Build history of the part. All positions in model axes, mm. Face numbers are marked on the shaded views. A direction names the side the tool comes from. Give positions to 0.01 mm unless a question says otherwise; leave off trailing zeros. Order: outer loops, then holes, each group sorted by start corner. A loop starts at its lowest first (then second) coordinate and runs counter-clockwise, first axis right, second up. Notation, with made-up numbers: (46, -39.5) -> (103, -39.5) arc R20 cw to (103, -24.5) -> close; hole circle Ø10 at (75.5, 61). An arc over 180 degrees is marked (long way). Write item = value, one per line. Start each with the question number.
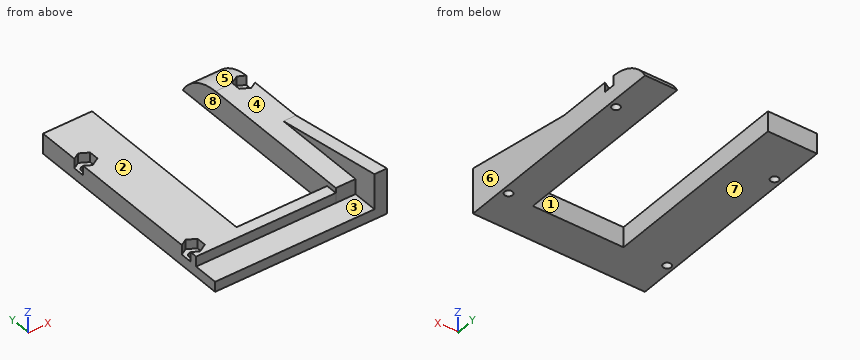
Autodesk Inventor part; units mm, degrees
ref_plane "Work Plane1" through (0, 0, 2.5241) normal (0, 0, 1) x (1, 0, 0)
ref_plane "YZ Plane" through (0, 0, 0) normal (1, 0, 0) x (0, 1, 0)
ref_plane "XZ Plane" through (0, 0, 0) normal (0, 1, 0) x (-1, 0, 0)
ref_plane "Work Plane1" through (0, 0, 2.5241) normal (0, 0, 1) x (1, 0, 0)
sketch "Sketch1" plane through (0, 0, 2.5241) normal (0, 0, 1) x (1, 0, 0)
  line L0 (-4, 272) -> (-4, -8) construction
  line L1 (4, 272) -> (4, -8) construction
  line L2 (76, 272) -> (76, -8) construction
  line L3 (84, 272) -> (84, -8) construction
  line L4 (84, -8) -> (-4, -8) construction
  line L5 (84, 106) -> (80, 106) construction
  line L6 (80, 110) -> (76, 110) construction
  line L7 (-3.365, 272) -> (-3.365, -7.365) construction
  line L8 (-3.365, -7.365) -> (83.365, -7.365) construction
  line L9 (83.365, -7.365) -> (83.365, 272) construction
  line L10 (-3.365, -7.365) -> (83.365, -7.365)
  line L11 (83.365, -7.365) -> (83.365, 107.95)
  line L12 (-3.365, 107.95) -> (-3.365, -7.365)
  circle A0 centre (0, 12) radius 2
  circle A1 centre (80, 12) radius 2
  circle A2 centre (0, 84) radius 2
  circle A3 centre (80, 84) radius 2
  line L13 (21.39, 107.95) -> (21.39, 11.177)
  line L14 (21.39, 11.177) -> (67.11, 11.177)
  line L15 (67.11, 11.177) -> (67.11, 107.95)
  line L16 (83.365, 107.95) -> (67.11, 107.95)
  line L17 (21.39, 107.95) -> (-3.365, 107.95)
  point P0 (0, 0)
  dimension "d0" = 0.635
  dimension "d1" = 8.89
  dimension "d2" = 45.72
  dimension "d18" = 18.542
extrude "Extrusion1" add sketch "Sketch1" along normal blind 10.16
sketch "Sketch2" plane through (0, 0, 12.6841) normal (0, 0, 1) x (1, 0, 0)
  line L0 (83.365, 107.95) -> (67.11, 107.95)
  line L1 (83.365, -7.365) -> (83.365, 107.95)
  line L2 (67.11, 107.95) -> (83.365, 107.95)
  line L3 (83.365, 107.95) -> (83.365, 23.8125)
  line L4 (67.11, 23.8125) -> (67.11, 107.95)
  circle A0 centre (80, 84) radius 2
  circle A1 centre (80, 84) radius 1.9939
  line L5 (83.365, 23.8125) -> (83.365, -7.365)
  line L6 (83.365, -7.365) -> (67.11, -7.365)
  line L7 (67.11, -7.365) -> (67.11, 23.8125)
  point P0 (0, 0)
  dimension "d5" = 3.9878
extrude "Extrusion2" add sketch "Sketch2" along normal blind 2.54 contours L1 L6 L7 L4 L0
fillet "Fillet1" radius 25.4 1 edges at (75.2375, 107.95, 15.2241)
sketch "Sketch3" plane through (0, 0, 12.6841) normal (0, 0, 1) x (1, 0, 0)
  circle A0 centre (0, 12) radius 2 construction
  circle A1 centre (0, 12) radius 4.8768 construction
  circle A2 centre (0, 84) radius 2 construction
  circle A3 centre (0, 84) radius 4.8768 construction
  circle A4 centre (80, 12) radius 2 construction
  line L0 (0, 16.8768) -> (4.2234, 14.4384)
  line L1 (4.2234, 14.4384) -> (4.2234, 9.5616)
  line L2 (4.2234, 9.5616) -> (0, 7.1232)
  line L3 (0, 7.1232) -> (-4.2234, 9.5616)
  line L4 (-4.2234, 9.5616) -> (-4.2234, 14.4384)
  line L5 (-4.2234, 14.4384) -> (0, 16.8768)
  line L6 (0, 88.8768) -> (4.2234, 86.4384)
  line L7 (4.2234, 86.4384) -> (4.2234, 81.5616)
  line L8 (4.2234, 81.5616) -> (0, 79.1232)
  line L9 (0, 79.1232) -> (-4.2234, 81.5616)
  line L10 (-4.2234, 81.5616) -> (-4.2234, 86.4384)
  line L11 (-4.2234, 86.4384) -> (0, 88.8768)
  point P0 (0, 0)
  dimension "d9" = 9.7536
  dimension "d10" = 9.7536
extrude "Extrusion3" cut sketch "Sketch3" against normal blind 4.826
sketch "Sketch4" plane through (0, 0, 15.2241) normal (0, 0, 1) x (1, 0, 0)
  circle A0 centre (80, 84) radius 2 construction
  circle A1 centre (80, 84) radius 4.8768 construction
  line L0 (80, 88.8768) -> (84.2234, 86.4384)
  line L1 (84.2234, 86.4384) -> (84.2234, 81.5616)
  line L2 (84.2234, 81.5616) -> (80, 79.1232)
  line L3 (80, 79.1232) -> (75.7766, 81.5616)
  line L4 (75.7766, 81.5616) -> (75.7766, 86.4384)
  line L5 (75.7766, 86.4384) -> (80, 88.8768)
  point P0 (0, 0)
  dimension "d14" = 9.7536
extrude "Extrusion4" cut sketch "Sketch4" against normal blind 4.826
sketch "Sketch5" plane through (0, 0, 12.6841) normal (0, 0, 1) x (1, 0, 0)
  line L0 (-3.365, -7.365) -> (67.11, -7.365)
  line L1 (-3.365, -7.365) -> (67.11, -7.365)
  line L2 (67.11, 5.335) -> (-3.365, 5.335)
  line L3 (-3.365, 5.335) -> (-3.365, -7.365)
  line L4 (67.11, 5.335) -> (67.11, -7.365)
  line L5 (-3.365, -7.365) -> (83.365, -7.365)
  point P0 (0, 0)
extrude "Extrusion5" cut sketch "Sketch5" against normal blind 5.08
sketch "Sketch13" plane through (83.365, -7.365, 15.2241) normal (1, 0, 0) x (0, 0, -1)
  line L0 (0, 0) -> (7.62, 0)
  line L1 (0, 0) -> (-10.16, 0)
  line L2 (0, 93.318) -> (0, 0)
  line L3 (0, 0) -> (0, 60.96)
  line L4 (0, 60.96) -> (-10.16, 0)
  point P0 (15.2241, 7.365)
  dimension "d54" = 10.16
  dimension "d55" = 60.96
extrude "Extrusion13" add sketch "Sketch13" against normal blind 6.35
sketch "Sketch14" plane through (0, 0, 15.2241) normal (0, 0, 1) x (1, 0, 0)
  line L0 (67.11, -7.365) -> (77.015, -7.365)
  line L1 (77.015, -7.365) -> (77.015, 53.595)
  line L2 (67.11, -7.365) -> (77.015, -7.365)
  line L3 (77.015, -7.365) -> (77.015, 5.3272)
  line L4 (77.015, 5.3272) -> (67.11, 5.3272)
  line L5 (67.11, 5.3272) -> (67.11, -7.365)
  point P0 (0, 0)
extrude "Extrusion14" cut sketch "Sketch14" against normal up to surface (7.62 mm away)
properties part number "Back Wall"
(1) Cut at B-B, the plane y = 84. Give the cut face in (x, z) (3 decimals), plus the area to 3 significant figures.
(2) Flat gauge pins, fed straight in: P1, Ø10, axis at x = 19.5, y = -0.5, coming from the +Z side; P2, Ø8, axis at x = 45.5, z = 5.5, coming from the +Y side; P3, Ø6, axis at x = 2, y = 13, coming from the +Z side. Where does each tip first touch, or does it go through?
(3) Wall check: line 1 (Y direction, x = 0, z = 4.8) (3 decimals); line 2 (X direction, y = 47, z = 9.75) (3 decimals); line 3 (Y direction, x = 80, z = 8.25) (3 decimals). Give the ranges that are in metal, low to high. Write a range as [from, to].
(4) Mould opens along X. For the marked faces 6, 7 and 8 say: released by +X, released by -X, zero draft, split by the parting line, or undercut.
(5) Cut at A-A, the plane y = 68. Give the cut face in (x, z) (3 decimals).
(6) Cut at C-C, the plane x = 45.5. Give the cut face in (y, z) (3 decimals), plus the area to 3 significant figures.
(7) 3-axis set-ups, long thin cutter, end or side, ignore diameter. For the marked faces 1, 2, 3, 4 and 5: which of +Z, -Z, +X, -X, +Y, -Y reach the whole face in a straight line?
(8) Cut at D-D, the plane z = 4.25. Give the cut face in (x, y) (3 decimals), plus the area to 3 significant figures.
Results:
q1.outline = (-3.365, 2.524) -> (-2, 2.524) -> (-2, 7.858) -> (-3.365, 7.858) -> close; (2, 2.524) -> (21.39, 2.524) -> (21.39, 12.684) -> (4.223, 12.684) -> (4.223, 7.858) -> (2, 7.858) -> close; (67.11, 2.524) -> (78, 2.524) -> (78, 10.398) -> (75.777, 10.398) -> (75.777, 15.224) -> (67.11, 15.224) -> close; (82, 2.524) -> (83.365, 2.524) -> (83.365, 10.398) -> (82, 10.398) -> close
q1.area = 332 mm2
q2.P1 = 7.6
q2.P2 = 11.18
q2.P3 = 12.68
q3.line_1 = [-7.365, 10], [14, 82], [86, 107.95]
q3.line_2 = [-3.365, 21.39], [67.11, 83.365]
q3.line_3 = [-7.365, 10], [14, 82], [86, 103.436]
q4.face_6 = released by +X
q4.face_7 = zero draft
q4.face_8 = undercut
q5.outline = (-3.365, 2.524) -> (21.39, 2.524) -> (21.39, 12.684) -> (-3.365, 12.684) -> close; (67.11, 2.524) -> (83.365, 2.524) -> (83.365, 15.224) -> (67.11, 15.224) -> close
q6.outline = (-7.365, 2.524) -> (11.177, 2.524) -> (11.177, 12.684) -> (5.335, 12.684) -> (5.335, 7.604) -> (-7.365, 7.604) -> close
q6.area = 124 mm2
q7.face_1 = +Z, -Z, +Y
q7.face_2 = +Z, -X, +Y, -Y
q7.face_3 = +Z, -X, -Y
q7.face_4 = +Z, -X, +Y
q7.face_5 = +Z, +X, +Y
q8.outline = (-3.365, -7.365) -> (83.365, -7.365) -> (83.365, 106.859) -> (67.11, 106.859) -> (67.11, 11.177) -> (21.39, 11.177) -> (21.39, 107.95) -> (-3.365, 107.95) -> close; hole circle Ø4 at (0, 12); hole circle Ø4 at (0, 84); hole circle Ø4 at (80, 12); hole circle Ø4 at (80, 84)
q8.area = 5,510 mm2
